Read the model definition and answer for the solid it produces. Units are mm, in the model's axes. Face numbers are marked on the shaded views. Coordinates: 2 decimals unless noted, no trailing zeros. Write each loop counter-clockwise with the first axis right and the second up, starting at its lowest first coordinate (ties: lowest second). Pieces come first, ordered by that corner, then holes.
(1) The part is cut by section C-C, the plane y = 8.5. Determine the outline of the cut face in (x, z), and give its area (3 significant figures).
(2) The part is cut by section D-D, the plane z = -7. Determine the outline of the cut face in (x, y).
(3) Straight lines are drawn through the part: line 1 along Z through (x, y) = (-14, 3.5); line 2 along X through (y, z) = (8.75, -1); line 3 along Z through (x, y) = (-12.75, 17.5). For each, find the intervals that lie inside material, in ascending order.
(4) Given pin 1 (2 mm diameter, centred on y = 12.5, z = 3.5, fed in from +X); pin 2 (6 mm diameter, centred on x = -10, z = -1.5, fed in from -Y); pin 3 (1.5 mm diameter, centred on y = 5, z = 2, fed in from -X); pin 4 (2 mm diameter, centred on y = 5, z = -6.5, fed in from -X), each flat-ended and moving along its own axis, determine where each tip first touches the part or whether it passes through.
(5) The part is cut by section B-B, the plane x = -12.25. Determine the outline of the cut face in (y, z), and give its area (3 significant figures).
(6) Determine the mould class of the marked faces 1, 2 and 3 for opening direction X: pulls with the +X half, pulls with the -X half, needs draft (parallel to the pull), parting line crosses it, or undercut.
(7) The part is cut by section A-A, the plane z = -1.75. Determine the outline of the cut face in (x, y).
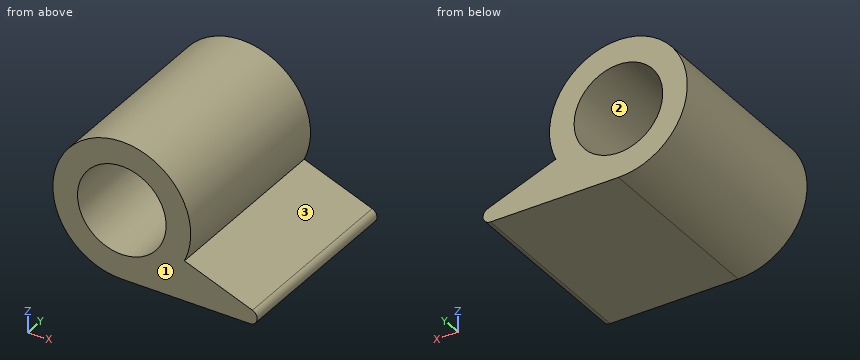
```python
from build123d import *

# Parameters (mm, degrees)
SALIENTE_EXTRUIR1_DEPTH = 19
CROQUIS3_R              = 4.5
CORTAR_EXTRUIR1_DEPTH   = 19


with BuildPart() as part:
    # Croquis2 → Saliente-Extruir1 (new body)
    with BuildSketch(Plane(origin=(0, 0, 0), x_dir=(1, 0, 0), z_dir=(0, 1, 0))):
        with BuildLine():
            Line((-13.873049235, 8.116898032), (-0.873049235, 8.116898032))
            ThreePointArc((-0.873049235, 8.116898032), (-0.135335411, 7.502095351), (-0.607084084, 6.665640205))
            Line((-0.607084084, 6.665640205), (-7.515172482, 4.045618436))
            ThreePointArc((-7.515172482, 4.045618436), (-17.647897389, -4.778059255), (-13.873049235, 8.116898032))
        make_face()
    extrude(amount=SALIENTE_EXTRUIR1_DEPTH)

    # Croquis3 → Cortar-Extruir1 (cut)
    with BuildSketch(Plane(origin=(0, 19, 0), x_dir=(1, 0, 0), z_dir=(0, 1, 0))):
        with Locations((-13.873049235, 1.116898032)):
            Circle(CROQUIS3_R)
    extrude(amount=-CORTAR_EXTRUIR1_DEPTH, mode=Mode.SUBTRACT)


solid = part.part
```
Computed:
1. outline: (-13.87, -8.12) - (-0.87, -8.12) arc R0.75 ccw to (-0.61, -6.67) - (-7.52, -4.05) arc R7 ccw (long way) to start; hole circle Ø9 at (-13.87, -1.12)
1. area: 117 mm2
2. outline: (-17.67, 0) - (-0.22, 0) - (-0.22, 19) - (-17.67, 19) - close
3. line 1: z = -8.12 to -5.62, 3.38 to 5.88
3. line 2: x = -20.87 to -18.37, -9.37 to -6.87
3. line 3: z = -8.12 to -5.47, 3.24 to 5.79
4. pin 1: stops at x = -7.88
4. pin 2: stops at y = 0
4. pin 3: stops at x = -20.46
4. pin 4: stops at x = -19.33
5. outline: (0, -8.12) - (19, -8.12) - (19, -5.31) - (0, -5.31) - close; (0, 3.08) - (19, 3.08) - (19, 5.69) - (0, 5.69) - close
5. area: 103 mm2
6. face 1: needs draft
6. face 2: undercut
6. face 3: pulls with the +X half
7. outline: (-20.84, 0) - (-18.33, 0) - (-18.33, 19) - (-20.84, 19) - close; (-9.42, 0) - (-6.9, 0) - (-6.9, 19) - (-9.42, 19) - close
